Verification items for the finished model (mm, model axes). A direction names the side the tool comes from. Round coordinates to 2 decimals unless told otherwise and drop trailing zeros. Write each loop counter-clockwise with the first axis right and the second up, starting at its lowest first coordinate (ties: lowest second). Pieces come first, ordered by that corner, then holes. Notation, with made-up numbers: (55, 56.25) - (99, 56.25) arc R17 ccw to (99, 78.25) - close; hole circle Ø1 at (69.5, 21). An arc over 180 degrees is marked (long way). Answer as a JSON object with one key per item and string values.
Autodesk Fusion 360 part; units mm, degrees
sketch "スケッチ1" plane through (0, 0, 0) normal (0, 0, 1) x (1, 0, 0)
  line L0 (7.5, 174.8326) -> (7.5, 25.1674)
  line L1 (0, 200) -> (0, 0)
  line L2 (0, 0) -> (80, 0)
  line L3 (80, 7.8285) -> (80, 0)
  line L4 (18.4541, 13.2131) -> (80, 7.8285)
  arc A0 (7.5, 25.1674) -> (18.4541, 13.2131) centre (19.5, 25.1674) ccw
  line L5 (80, 192.1715) -> (18.4541, 186.7869)
  line L6 (0, 200) -> (80, 200)
  arc A1 (18.4541, 186.7869) -> (7.5, 174.8326) centre (19.5, 174.8326) ccw
  line L7 (80, 200) -> (80, 192.1715)
extrude "押し出し1" add sketch "スケッチ1" along normal blind 100
Q1. Section check C-C, the plane y = 96.5. Record the cut outline in (x, z), then the cut area to 3 significant figures.
Geometry check:
{"outline": "(0, 0) - (7.5, 0) - (7.5, 100) - (0, 100) - close", "area": "750 mm2"}
Q2. Section check B-B, the plane z = 71. Record the cut outline in (x, y).
Geometry check:
{"outline": "(0, 0) - (80, 0) - (80, 7.83) - (18.45, 13.21) arc R12 cw to (7.5, 25.17) - (7.5, 174.83) arc R12 cw to (18.45, 186.79) - (80, 192.17) - (80, 200) - (0, 200) - close"}
Q3. Section check A-A, the plane x = 67. Record the cut outline in (y, z).
Geometry check:
{"outline": "(0, 0) - (8.97, 0) - (8.97, 100) - (0, 100) - close; (191.03, 0) - (200, 0) - (200, 100) - (191.03, 100) - close"}
Q4. Set-up check for faces 5 (the flat face through (0, 101, 49)), 6 (the cylindrical face through (10.57, 182.85, 49.3)): record each of +Z, -Z, +X, -X, +Y, -Y from which the full face is reachable in a straight line by a thin tool's end or side.
Geometry check:
{"face 5": "+Z, -Z, -X, +Y, -Y", "face 6": "+Z, -Z, +X"}
Q5. Gauge pin test, flat end, axial feed: P1, Ø10, axis at y = 164, z = 85.5, coming from the +X side. Record the tip position at first contact, or that the pin passes through.
Geometry check:
{"P1": "stops at x = 7.5"}
Q6. Material ranges on line 1 along X through (y, z) = (149, 16.5); line 2 along Y through (x, z) = (28.5, 59); line 3 along Y through (x, z) = (69.5, 77), recorded low to high. Write a range as [from, to].
Geometry check:
{"line 1": "x = [0, 7.5]", "line 2": "y = [0, 12.33], [187.67, 200]", "line 3": "y = [0, 8.75], [191.25, 200]"}
Q7. Section check D-D, the plane x = 57. Record the cut outline in (y, z).
Geometry check:
{"outline": "(0, 0) - (9.84, 0) - (9.84, 100) - (0, 100) - close; (190.16, 0) - (200, 0) - (200, 100) - (190.16, 100) - close"}
Q8. Release check for a two-part mould opening along Y. For faces 1 (the cylindrical face through (10.737, 16.969, 49.3)), 2 (the flat face through (80, 4, 49)), 3 (the flat face through (48.8, 10.56, 49.3)), 4 (the flat face through (39, 0, 49)) record: released by +Y, released by -Y, zero draft, split by the parting line, or undercut.
Geometry check:
{"face 1": "undercut", "face 2": "zero draft", "face 3": "undercut", "face 4": "released by -Y"}
